Design review of the part built by this model. Coordinates are the model's own, in mm. Coordinates: 2 decimals unless noted, no trailing zeros. Loops run counter-clockwise (first coordinate to the right, second up) from the corner with the lowest first, then second, coordinate; pieces in that order, holes last. Notation, with made-up numbers: (-19.5, 52) -> (34.5, 52) arc R21 ccw to (34.5, 56) -> close; hole circle Ø1 at (40, -9.75). An arc over 180 degrees is marked (long way). Use a Markdown table: item, result. Add a question column.
Q1. Take a section at C-C on x = 89.5. Write out the cut boundary in (y, z), plus the area to 3 significant figures.
Q2. Take a section at B-B on y = -7. Write out the cut boundary in (x, z), plus the area to 3 significant figures.
Q3. For probe 1 along X at (y, z) = (-57, 1.45); probe 2 along X at (y, z) = (-59.5, 1.8); probe 3 along X at (y, z) = (11.5, 1.1), list the stretches that pass through material, from the lowest coordinate up.
Q4. Take a section at A-A on z = 0.85. Write out the cut boundary in (x, y) (3 decimals).
from build123d import *

# Parameters (mm, degrees)
BOSS_EXTRUDE1_DEPTH = 2.54
SKETCH2_R           = 3.175
CUT_EXTRUDE1_DEPTH  = 252.765490419


with BuildPart() as part:
    # Sketch1 → Boss-Extrude1 (new body)
    with BuildSketch(Plane.XY):
        with BuildLine():
            Line((56.475591943, 100.965617501), (70.541585889, 126.112441388))
            Line((70.541585889, 126.112441388), (121.527407416, 97.59328286))
            Line((121.527407416, 97.59328286), (35.036266464, -57.033364763))
            ThreePointArc((35.036266464, -57.033364763), (23.451402169, -68.229473927), (7.610684951, -71.167776012))
            Line((7.610684951, -71.167776012), (-217.887729561, -69.42085916))
            Line((-217.887729561, -69.42085916), (-217.887729561, 54.938377315))
            Line((-217.887729561, 54.938377315), (-189.368571032, 105.924198843))
            Line((-189.368571032, 105.924198843), (-150.227007979, 84.030181873))
            Line((-150.227007979, 84.030181873), (56.475591943, 100.965617501))
        make_face()
    extrude(amount=BOSS_EXTRUDE1_DEPTH)

    # Sketch2 → Cut-Extrude1 (cut, through all)
    with BuildSketch(Plane.XY.offset(2.54)):
        with BuildLine():
            ThreePointArc((-0.387630151, -36.96777295), (-1.317566121, -34.72270892), (-3.562630151, -33.79277295))
            Line((-3.562630151, -33.79277295), (-3.562630151, -40.14277295))
            ThreePointArc((-3.562630151, -40.14277295), (-1.317566121, -39.212836981), (-0.387630151, -36.96777295))
        make_face()
        with BuildLine():
            Line((-3.562630151, -40.14277295), (-3.562630151, -33.79277295))
            ThreePointArc((-3.562630151, -33.79277295), (-6.737630151, -36.96777295), (-3.562630151, -40.14277295))
        make_face()
        with Locations((-54.362630151, 75.80822705)):
            Circle(SKETCH2_R)
        with Locations((-105.162630151, -62.36777295)):
            Circle(SKETCH2_R)
    extrude(amount=-CUT_EXTRUDE1_DEPTH, mode=Mode.SUBTRACT)


solid = part.part
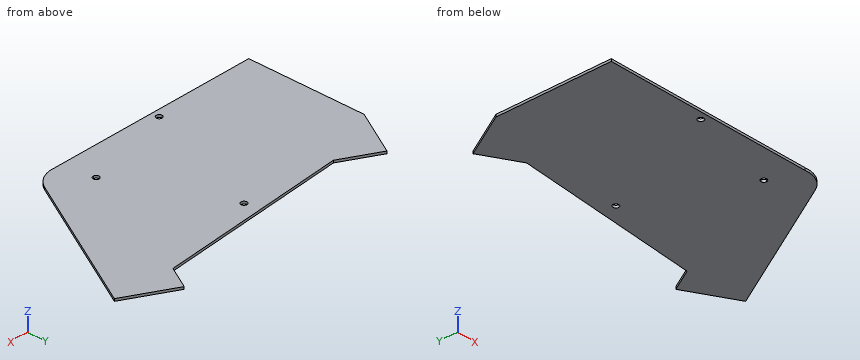
Answer list:
| question | item | result |
|---|---|---|
| 1 | outline | (40.34, 0) -> (115.51, 0) -> (115.51, 2.54) -> (40.34, 2.54) -> close |
| 1 | area | 191 mm² |
| 2 | outline | (-217.89, 0) -> (63.02, 0) -> (63.02, 2.54) -> (-217.89, 2.54) -> close |
| 2 | area | 714 mm² |
| 3 | probe 1 | -217.89 to 35.05 |
| 3 | probe 2 | -217.89 to -106.53, -103.8 to 33.48 |
| 3 | probe 3 | -217.89 to 73.37 |
| 4 | outline | (-217.888, -69.421) -> (7.611, -71.168) arc R27.94 ccw to (35.036, -57.033) -> (121.527, 97.593) -> (70.542, 126.112) -> (56.476, 100.966) -> (-150.227, 84.03) -> (-189.369, 105.924) -> (-217.888, 54.938) -> close; hole circle Ø6.35 at (-105.163, -62.368); hole circle Ø6.35 at (-54.363, 75.808); hole circle Ø6.35 at (-3.563, -36.968) |
